Study the drawing (mm; zero at the part's minimum x, y, z) and answer. A direction names the side the tool comes from. Give positions to 0.01 mm unless a question says otherwise; leave off trailing zeros. Order: outer loops, then holes, each group sorted by start corner. A loop starts at its lowest first (then second) coordinate and runs counter-clockwise, first axis right, second up. Notation, with made-up numbers: (16, 1.25) - (68, 1.25) arc R20 ccw to (68, 28.25) - close; hole circle Ø10 at (18.25, -19). An arc over 180 degrees is marked (long way). Write each question's results on one line, items separated by ' | '. Start each with the question number.
1. Section C-C (x = 18) is taken. Give the vertices of the cut face in (y, z), and give its area (3 significant figures).
2. Flat-ended cylindrical pins translate along their axes: pin 1 (1.9 mm diameter, centred on x = 37, y = 4.5, fed in from +Z); pin 2 (3 mm diameter, centred on y = 3.5, z = 4.5, fed in from -X); pin 3 (3 mm diameter, centred on y = 3.5, z = 26, fed in from +X). Find the tip coordinate at first contact, or state that the pin passes through.
3. Find the intervals of material crossed by L1, parallel to X at y = 1.5, z = 19; L2, parallel to Z at x = 11, y = 6; L3, parallel to Z at x = 26, y = 2.5, in increasing order.
4. Which of the six approach directions +Z, -Z, +X, -X, +Y, -Y give full straight-line access (tool end or side, diameter ignored) to the marked faces 5, 6, 7, 8 and 9?
5. Section D-D (x = 5) is taken. Give the vertices of the cut face in (y, z), and give its area (3 significant figures).
6. Section B-B (y = 2.75) is taken. Give the vertices of the cut face in (x, z), and give its area (3 significant figures).
7. Section A-A (z = 14.25) is taken. Give the vertices of the cut face in (x, y).
8. Determine the mould class of the marked faces 1, 2, 3 and 4 for opening direction X: released by +X, released by -X, zero draft, split by the parting line, or undercut.
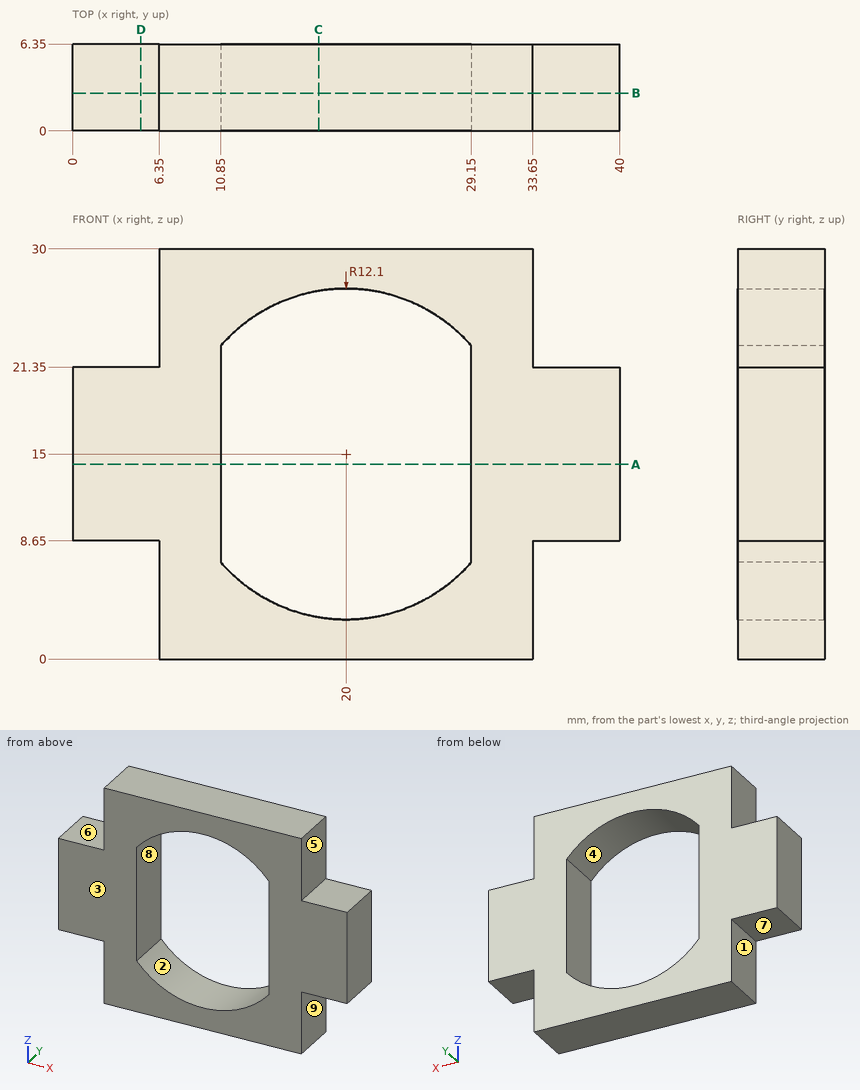
Reported:
1) outline: (0, 0) - (6.35, 0) - (6.35, 3.07) - (0, 3.07) - close; (0, 26.93) - (6.35, 26.93) - (6.35, 30) - (0, 30) - close | area: 38.9 mm²
2) pin 1: z = 21.35 | pin 2: x = 6.35 | pin 3: x = 33.65
3) L1: 0 to 10.85, 29.15 to 40 | L2: 0 to 6.91, 23.09 to 30 | L3: 0 to 4.49, 25.51 to 30
4) face 5: +Z, +X, +Y, -Y | face 6: +Z, -X, +Y, -Y | face 7: -Z, -X, +Y, -Y | face 8: +Y, -Y | face 9: -Z, +X, +Y, -Y
5) outline: (0, 8.65) - (6.35, 8.65) - (6.35, 21.35) - (0, 21.35) - close | area: 80.6 mm²
6) outline: (0, 8.65) - (6.35, 8.65) - (6.35, 0) - (33.65, 0) - (33.65, 8.65) - (40, 8.65) - (40, 21.35) - (33.65, 21.35) - (33.65, 30) - (6.35, 30) - (6.35, 21.35) - (0, 21.35) - close; hole (10.85, 7.08) arc R12.1 ccw to (29.15, 7.08) - (29.15, 22.92) arc R12.1 ccw to (10.85, 22.92) - close | area: 584 mm²
7) outline: (0, 0) - (10.85, 0) - (10.85, 6.35) - (0, 6.35) - close; (29.15, 0) - (40, 0) - (40, 6.35) - (29.15, 6.35) - close
8) face 1: released by -X | face 2: undercut | face 3: zero draft | face 4: undercut
